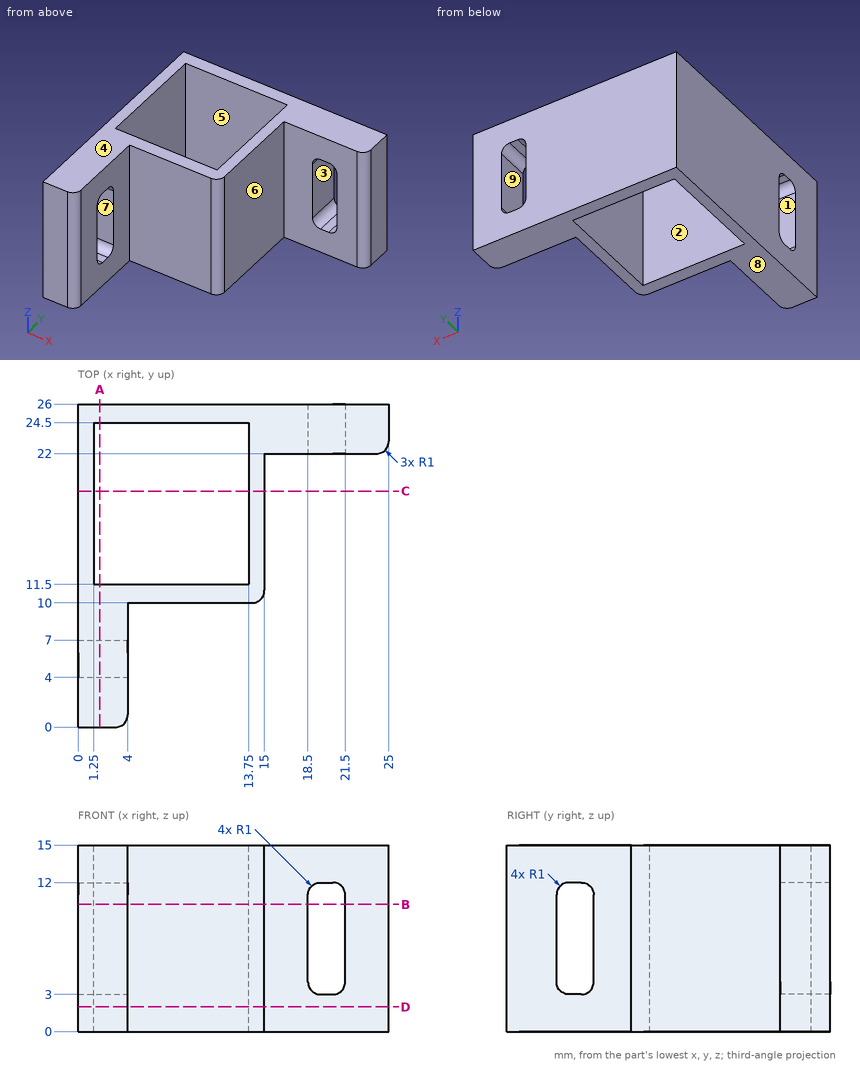
Design review of the part shown in the three views and the two pictorial views. Dimensions are in mm from the part's minimum x, y and z. A direction names the side the tool comes from. Give positions to 0.01 mm unless a question says otherwise; leave off trailing zeros. Loops run counter-clockwise (first coordinate to the right, second up) from the corner with the lowest first, then second, coordinate; pieces in that order, holes last. Notation, with made-up numbers: M -19,48 L 30,48 A20 ccw 30,60 Z; hole C 12,58 d8. An arc over 180 degrees is marked long. Answer as a JSON object with one key per item and string values. Group by question number.
Q1. For probe 1 along Y at (x, z) = (2.5, 9.5); probe 2 along X at (y, z) = (14, 9); probe 3 along X at (y, z) = (22.5, 6), list the stretches that pass through material, from the lowest coordinate up. Write a range as [from, to].
Q2. Add section A-A on x = 1.75. Give the boundary of the cut face in (y, z).
Q3. Add section D-D on z = 2. Give the boundary of the cut face in (x, y).
Q4. Add section B-B on z = 10.25. Give the boundary of the cut face in (x, y).
Q5. Insertion check: P1, Ø4, axis at x = 22, z = 11, coming from the -Y side; P2, Ø4.5, axis at y = 5, z = 6, coming from the +X side; P3, Ø1, axis at x = 12.5, y = 21, coming from the -Z side; P4, Ø8, axis at x = 17.5, z = 13.5, coming from the -Y side. Each pin has a flat end and moves straight along its axis. Give the tip position at first contact, or say it passes through.
Q6. Mouldability with a two-part tool opening along Z and no side actions: class the marked faces 1, 2, 3 and 4 as +Z half, -Z half, draft (parallel to the pull), parting line (faces both ways), or undercut.
Q7. Add section C-C on y = 19. Give the boundary of the cut face in (x, z).
Q8. Tool access review of the marked faces 5, 6, 7, 8 and 9: name each direction out of +Z, -Z, +X, -X, +Y, -Y from which nothing blocks a thin tool from reaching the whole face with its end or side.
Checked values:
{
 "1": {"probe 1": "[0, 4], [7, 11.5], [24.5, 26]", "probe 2": "[0, 1.25], [13.75, 15]", "probe 3": "[0, 1.25], [13.75, 18.5], [21.5, 24.87]"},
 "2": {"outline": "M 0,0 L 11.5,0 L 11.5,15 L 0,15 Z; M 24.5,0 L 26,0 L 26,15 L 24.5,15 Z; hole M 4,4 A1 ccw 5,3 L 6,3 A1 ccw 7,4 L 7,11 A1 ccw 6,12 L 5,12 A1 ccw 4,11 Z"},
 "3": {"outline": "M 0,0 L 3,0 A1 ccw 4,1 L 4,10 L 14,10 A1 ccw 15,11 L 15,22 L 24,22 A1 ccw 25,23 L 25,26 L 0,26 Z; hole M 1.25,11.5 L 13.75,11.5 L 13.75,24.5 L 1.25,24.5 Z"},
 "4": {"outline": "M 0,0 L 3,0 A1 ccw 4,1 L 4,4 L 0,4 Z; M 0,7 L 4,7 L 4,10 L 14,10 A1 ccw 15,11 L 15,22 L 18.5,22 L 18.5,26 L 0,26 Z; M 21.5,22 L 24,22 A1 ccw 25,23 L 25,26 L 21.5,26 Z; hole M 1.25,11.5 L 13.75,11.5 L 13.75,24.5 L 1.25,24.5 Z"},
 "5": {"P1": "y = 22", "P2": "x = 4", "P3": "through", "P4": "y = 10"},
 "6": {"face 1": "undercut", "face 2": "draft", "face 3": "undercut", "face 4": "+Z half"},
 "7": {"outline": "M 0,0 L 1.25,0 L 1.25,15 L 0,15 Z; M 13.75,0 L 15,0 L 15,15 L 13.75,15 Z"},
 "8": {"face 5": "+Z, -Z", "face 6": "+Z, -Z, +X, -Y", "face 7": "+X, -X", "face 8": "-Z, +X, -X, +Y, -Y", "face 9": "+Y, -Y"}
}
